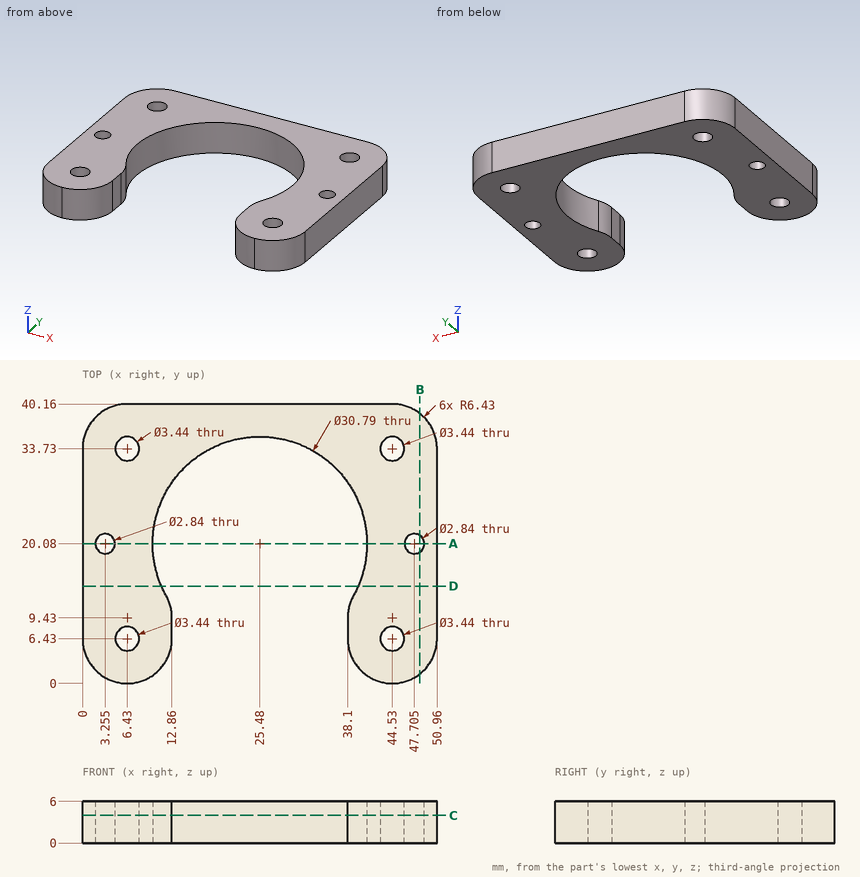
The drawing under review shows one solid part. Ordinate dimensions are in mm from its lowest x, y, z. Coordinates: 2 decimals unless noted, no trailing zeros. Write each loop counter-clockwise with the first axis right and the second up, starting at its lowest first coordinate (ties: lowest second). Pieces come first, ordered by that corner, then holes. Notation, with made-up numbers: (64, 61) - (110, 61) arc R17 ccw to (110, 94) - close; hole circle Ø9 at (76, 0.5). An arc over 180 degrees is marked (long way). Use one line per item in the form item = value.
Q1. For probe 1 along Y at (x, z) = (7, 1.55) (1 decimal); probe 2 along Y at (x, z) = (46, 3.5) (1 decimal); probe 3 along X at (y, z) = (13, 2.05), list the stretches that pass through material, from the lowest coordinate up.
Taken from the geometry:
probe_1 = 0 to 4.8, 8.1 to 32.1, 35.4 to 40.2
probe_2 = 0.2 to 5.5, 7.3 to 32.8, 34.6 to 40
probe_3 = 0 to 11.81, 39.15 to 50.96
Q2. Insertion check: pin 1 Ø2 at (x, z) = (29.5, 1) entering from -Y. The pin has a flat end and moves straight along its axis. Give the tip position at first contact, or say it passes through.
Taken from the geometry:
pin_1 = 34.63
Q3. Consider section A-A (y = 20.08). Write out the cut boundary in (x, z) (1 decimal).
Taken from the geometry:
outline = (0, 0) - (1.8, 0) - (1.8, 6) - (0, 6) - close; (4.7, 0) - (10.1, 0) - (10.1, 6) - (4.7, 6) - close; (40.9, 0) - (46.3, 0) - (46.3, 6) - (40.9, 6) - close; (49.1, 0) - (51, 0) - (51, 6) - (49.1, 6) - close
Q4. Consider section D-D (y = 14). Write out the cut boundary in (x, z).
Taken from the geometry:
outline = (0, 0) - (11.34, 0) - (11.34, 6) - (0, 6) - close; (39.62, 0) - (50.96, 0) - (50.96, 6) - (39.62, 6) - close
Q5. Consider section C-C (z = 4). Count the separate pieces of the cut face and the enclosed holes in it, plus the area to 3 significant figures.
Taken from the geometry:
separate_pieces = 1
enclosed_holes = 6
area = 1,030 mm^2
Q6. Consider section B-B (x = 48.5). Write out the cut boundary in (y, z), plus the area to 3 significant figures.
Taken from the geometry:
outline = (1.37, 0) - (18.9, 0) - (18.9, 6) - (1.37, 6) - close; (21.26, 0) - (38.79, 0) - (38.79, 6) - (21.26, 6) - close
area = 210 mm^2
